Autodesk Inventor part; units mm, degrees
ref_plane "YZ Plane" through (0, 0, 0) normal (1, 0, 0) x (0, 1, 0)
ref_plane "XZ Plane" through (0, 0, 0) normal (0, 1, 0) x (-1, 0, 0)
ref_plane "XY Plane" through (0, 0, 0) normal (0, 0, 1) x (1, 0, 0)
sketch "Sketch1" plane through (0, 0, 0) normal (1, 0, 0) x (0, 1, 0)
  line L0 (2.5, 2.81) -> (2.5, 11.31)
  spline S0 degree 2 poles (-3.9658, 2.81) (-4.0258, 2.8689) (-4.0876, 2.9295) knots 0 0 0 0.017848 0.017848 0.017848 weights 1 1.00044 1.00066
  line L1 (-2.5, 11.31) -> (-2.5, 2.81)
  line L2 (1.7321, 14.76) -> (1.7821, 14.81)
  line L3 (-1.7821, 14.81) -> (4.1614, 14.81)
  arc A0 (4.1614, 13.31) -> (4.1614, 14.81) centre (3.5, 14.06) ccw
  line L4 (4.1614, 13.31) -> (2.5, 13.31)
  line L5 (2.5, 13.31) -> (2.5, -11.19)
  line L6 (2.5, -11.19) -> (2, -11.69)
  line L7 (2, -11.69) -> (-2, -11.69)
  line L8 (-2, -11.69) -> (-2.5, -11.19)
  line L9 (-2.5, -11.19) -> (-2.5, 13.31)
  line L10 (-2.5, 13.31) -> (-4.1614, 13.31)
  arc A1 (-4.1614, 14.81) -> (-4.1614, 13.31) centre (-3.5, 14.06) ccw
  line L11 (-4.1614, 14.81) -> (-1.7821, 14.81)
  line L12 (-1.7821, 14.81) -> (-1.7321, 14.76)
  line L13 (-2, -11.69) -> (2, -11.69)
  line L14 (0, -11.69) -> (0, 14.81)
  point P0 (0, 0)
revolve "Revolution1" add sketch "Sketch1" angle 360 about axis through (0, 0, -11.69) along (0, 0, 1) contours L5 L6 L7 L14 L3 A0 L4 L0
sketch "Sketch2" plane through (0, 0, 14.81) normal (0, 0, 1) x (1, 0, 0)
  line L0 (1.732, 0) -> (0.866, -1.5)
  line L1 (0.866, -1.5) -> (-0.866, -1.5)
  line L2 (-0.866, -1.5) -> (-1.732, 0)
  line L3 (-1.732, 0) -> (-0.866, 1.5)
  line L4 (-0.866, 1.5) -> (0.866, 1.5)
  line L5 (0.866, 1.5) -> (1.732, 0)
  point P0 (0, 0)
  point P1 (0, 0)
  dimension "d1" = 3.464
extrude "Extrusion1" cut sketch "Sketch2" against normal blind 2.3
sketch "Sketch3" plane through (0, 0, 0) normal (0, 1, 0) x (-1, 0, 0)
  line L0 (0.866, 14.81) -> (-0.866, 14.81)
  line L1 (0.866, 14.81) -> (0.866, 12.51)
  line L2 (0.866, 12.51) -> (-0.866, 12.51)
  line L3 (-0.866, 14.81) -> (-0.866, 12.51)
  line L4 (1.732, 14.81) -> (1.732, 12.51)
  circle A0 centre (0, 19.6597) radius 5.1497
  line L5 (0, 14.81) -> (0, 14.51)
  line L6 (0, 14.81) -> (0, 24.8094)
  point P0 (0, 0)
  dimension "d5" = 0.3
revolve "Revolution2" cut sketch "Sketch3" angle 360 about axis through (0, 0, 14.81) along (0, 0, 1) contours L5 A0 L3 L0 | L0 L3 A0 L6
thread "Thread1"
properties part number "Low Profile Screw M5 [25mm]" material "Steel"
Could you check a few things on this model? Use its own coordinates, in mm. A direction names the side the tool comes from. Give positions to 0.01 mm unless a question says otherwise; leave off trailing zeros. Loops run counter-clockwise (first coordinate to the right, second up) from the corner with the lowest first, then second, coordinate; pieces in that order, holes last. Notation, with made-up numbers: (-14, 19) -> (8, 19) arc R28 ccw to (8, 46) -> close; hole circle Ø11 at (-27, 12). An arc over 180 degrees is marked (long way). Return JSON: item names as keys, results as strings.
Item 1: If we section it at A-A on x = 0: List the corners of the cut face in (y, z) for me, plus the area to 3 significant figures.
Geometry results:
{"outline": "(-4.16, 13.31) -> (-2.5, 13.31) -> (-2.5, -11.19) -> (-2, -11.69) -> (2, -11.69) -> (2.5, -11.19) -> (2.5, 13.31) -> (4.16, 13.31) arc R1 ccw to (4.16, 14.81) -> (1.73, 14.81) arc R5.15 cw to (1.5, 14.73) -> (1.5, 12.51) -> (-1.5, 12.51) -> (-1.5, 14.73) arc R5.15 cw to (-1.73, 14.81) -> (-4.16, 14.81) arc R1 ccw to start", "area": "131 mm²"}
Item 2: Which directions (+Z, -Z, +X, -X, +Y, -Y) give clear straight access to the entire face, cutting with the end or side of a thin tool? Please do faces 4 (the flat face through (0, 0, -11.69)), 5 (the flat face through (1.293, 0.761, 13.676)), 6 (the flat face through (2, 2, 13.31)).
Geometry results:
{"face 4": "-Z, +X, -X, +Y, -Y", "face 5": "+Z", "face 6": "-Z"}
Item 3: I need wall thicknesses on L1, parallel to Z at x = -2.5, y = 1.5; L2, parallel to Z at x = 0.25, y = 0.5; L3, parallel to Y at x = 1.25, z = -1.5. Which ranges of each line are inside material? Lowest first, please. Write a range as from..to.
Geometry results:
{"L1": "z = 13.31..14.81", "L2": "z = -11.69..12.51", "L3": "y = -2.17..2.17"}
Item 4: We'd pull the mould along Y, two halves only. Please class faces 1 (the cylindrical face through (-2.44, -0.54, 0.89)), 2 (the flat face through (2, 0, 14.81)), 3 (the flat face through (1.305, -0.739, 13.676)): +Y half, -Y half, draft (parallel to the pull), parting line (faces both ways), or undercut.
Geometry results:
{"face 1": "parting line", "face 2": "draft", "face 3": "undercut"}
Item 5: If we section it at B-B on z = 0.5: List the corners of the cut face in (x, y) for me, plus the area to 3 significant figures.
Geometry results:
{"outline": "circle Ø5 at (0, 0)", "area": "19.6 mm²"}
Item 6: I'm going to push flat-ended pins straight in: pin 1 (1 mm diameter, centred on x = -1, z = -3, fed in from -Y); pin 2 (0.5 mm diameter, centred on x = 0, z = 13.5, fed in from -Y); pin 3 (1 mm diameter, centred on x = 0, z = -1.5, fed in from +Y). Where does each tip first touch, or does it pass through?
Geometry results:
{"pin 1": "stops at y = -2.45", "pin 2": "stops at y = -4.45", "pin 3": "stops at y = 2.5"}
